```python
from build123d import *

# Parameters (mm, degrees)
SKETCH1_W           = 32
SKETCH1_H           = 15
BOSS_EXTRUDE1_DEPTH = 10
SKETCH2_R           = 2.5
BOSS_EXTRUDE2_DEPTH = 2
SKETCH3_W           = 30
SKETCH3_H           = 13
CUT_EXTRUDE1_DEPTH  = 9
SKETCH4_R           = 3.5
SKETCH4_R_2         = 3
BOSS_EXTRUDE3_DEPTH = 9
BOSS_EXTRUDE4_DEPTH = 7


with BuildPart() as part:
    # Sketch1 → Boss-Extrude1 (new body)
    with BuildSketch(Plane(origin=(0, 0, 0), x_dir=(1, 0, 0), z_dir=(0, 1, 0))):
        Rectangle(SKETCH1_W, SKETCH1_H)
    extrude(amount=BOSS_EXTRUDE1_DEPTH)

    # Sketch2 → Boss-Extrude2 (add)
    with BuildSketch(Plane(origin=(0, 10, 0), x_dir=(1, 0, 0), z_dir=(0, 1, 0))):
        with Locations((-12, -3.5)):
            Circle(SKETCH2_R)
        with Locations((-4, -3.5)):
            Circle(SKETCH2_R)
        with Locations((4, -3.5)):
            Circle(SKETCH2_R)
        with Locations((12, -3.5)):
            Circle(SKETCH2_R)
        with Locations((12, 3.5)):
            Circle(SKETCH2_R)
        with Locations((4, 3.5)):
            Circle(SKETCH2_R)
        with Locations((-4, 3.5)):
            Circle(SKETCH2_R)
        with Locations((-12, 3.5)):
            Circle(SKETCH2_R)
    extrude(amount=BOSS_EXTRUDE2_DEPTH)

    # Sketch3 → Cut-Extrude1 (cut)
    with BuildSketch(Plane.XZ):
        Rectangle(SKETCH3_W, SKETCH3_H)
    extrude(amount=-CUT_EXTRUDE1_DEPTH, mode=Mode.SUBTRACT)

    # Sketch4 → Boss-Extrude3 (add)
    with BuildSketch(Plane.XZ.offset(-9)):
        Circle(SKETCH4_R)
        Circle(SKETCH4_R_2, mode=Mode.SUBTRACT)
        with Locations((8, 0)):
            Circle(SKETCH4_R)
        with Locations((8, 0)):
            Circle(SKETCH4_R_2, mode=Mode.SUBTRACT)
        with Locations((-8, 0)):
            Circle(SKETCH4_R)
        with Locations((-8, 0)):
            Circle(SKETCH4_R_2, mode=Mode.SUBTRACT)
    extrude(amount=BOSS_EXTRUDE3_DEPTH)

    # Sketch5 → Boss-Extrude4 (add)
    with BuildSketch(Plane.XZ.offset(-9)):
        with BuildLine():
            Line((-0.272235441, -6.5), (0.272235441, -6.5))
            Line((0.272235441, -6.5), (0.272235441, -3.48939649))
            ThreePointArc((0.272235441, -3.48939649), (0, -3.5), (-0.272235441, -3.48939649))
            Line((-0.272235441, -3.48939649), (-0.272235441, -6.5))
        make_face()
        with BuildLine():
            Line((-0.272235441, 6.5), (0.272235441, 6.5))
            Line((0.272235441, 6.5), (0.272235441, 3.48939649))
            ThreePointArc((0.272235441, 3.48939649), (0, 3.5), (-0.272235441, 3.48939649))
            Line((-0.272235441, 3.48939649), (-0.272235441, 6.5))
        make_face()
    extrude(amount=BOSS_EXTRUDE4_DEPTH)


solid = part.part
```
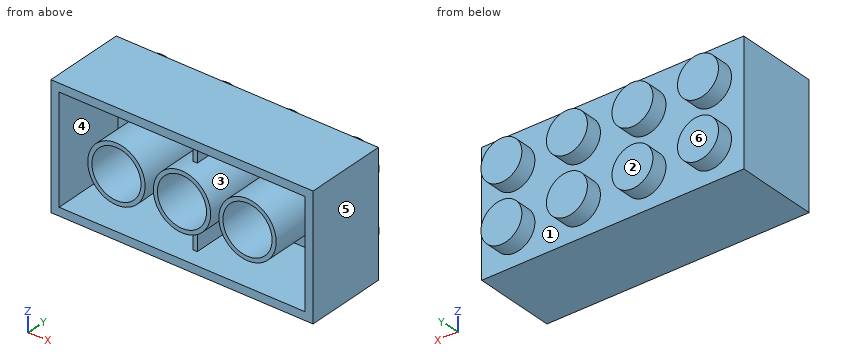
Geometry check sheet. Reference: the model listing, model coordinates, mm. Face numbers are marked on the shaded views. A direction names the side the tool comes from. Give positions to 0.01 mm unless a question says otherwise; leave off trailing zeros. Order: outer loops, then holes, each group sorted by start corner. A loop starts at its lowest first (then second) coordinate and runs counter-clockwise, first axis right, second up. Notation, with made-up numbers: (-32.75, -12.5) - (-5.75, -12.5) arc R31 ccw to (-5.75, 24.5) - close; hole circle Ø3 at (32, 35.5). An arc over 180 degrees is marked (long way). Answer in a Markdown table with one row per item. Add a question column.
Q1. Cross-section at C-C, the plane x = 8. Enter the section's corners in (y, z), then the cut area to 3 significant figures.
Q2. Material ranges on probe 1 along Z at (x, y) = (-8, 5.75); probe 2 along X at (y, z) = (3.75, 4.25); probe 3 along X at (y, z) = (11, 4), recorded low to high. Write a range as from..to.
Q3. Mould release check, pull along X, two halves, no side actions. Record for the marked faces 4, 5 and 6: pulls with the +X half, pulls with the -X half, needs draft (parallel to the pull), parting line crosses it, or undercut.
Q4. Cross-section at A-A, the plane y = 2.5. Enter the section's corners in (x, z), then the cut area to 3 significant figures.
Q5. Gauge pin test, flat ends, axial feed: pin 1 (0.6 mm diameter, centred on x = 0, z = -5, fed in from -Y); pin 2 (3 mm diameter, centred on x = -9, z = -3, fed in from +Y); pin 3 (1.8 mm diameter, centred on x = 8.5, z = -1, fed in from -Y); pin 4 (2 mm diameter, centred on x = 7, z = 5.5, fed in from +Y). Record the tip position at first contact, or that the pin passes through.
Q6. Cross-section at D-D, the plane x = 12. Enter the section's corners in (y, z), then the cut area to 3 significant figures.
Q7. Tool access check on the marked faces 1, 2 and 3. Record the directions out of +Z, -Z, +X, -X, +Y, -Y that give a thin tool (end or side, any length) a straight path to the whole face; none if there is none.
Check values:
| question | item | result |
|---|---|---|
| 1 | outline | (0, -7.5) - (10, -7.5) - (10, 7.5) - (0, 7.5) - (0, 6.5) - (9, 6.5) - (9, 3.5) - (0, 3.5) - (0, 3) - (9, 3) - (9, -3) - (0, -3) - (0, -3.5) - (9, -3.5) - (9, -6.5) - (0, -6.5) - close |
| 1 | area | 42.0 mm^2 |
| 2 | probe 1 | z = -7.5..-6.5, -3.5..-3, 3..3.5, 6.5..7.5 |
| 2 | probe 2 | x = -16..-15, -0.27..0.27, 15..16 |
| 2 | probe 3 | x = -14.45..-9.55, -6.45..-1.55, 1.55..6.45, 9.55..14.45 |
| 3 | face 4 | undercut |
| 3 | face 5 | pulls with the +X half |
| 3 | face 6 | needs draft |
| 4 | outline | (-16, -7.5) - (16, -7.5) - (16, 7.5) - (-16, 7.5) - close; circle Ø7 at (-8, 0); circle Ø7 at (8, 0); hole (-15, -6.5) - (-0.27, -6.5) - (-0.27, -3.49) arc R3.5 cw to (-0.27, 3.49) - (-0.27, 6.5) - (-15, 6.5) - close; hole circle Ø6 at (-8, 0); hole circle Ø6 at (0, 0); hole (0.27, -6.5) - (15, -6.5) - (15, 6.5) - (0.27, 6.5) - (0.27, 3.49) arc R3.5 cw to (0.27, -3.49) - close; hole circle Ø6 at (8, 0) |
| 4 | area | 124 mm^2 |
| 5 | pin 1 | stops at y = 2 |
| 5 | pin 2 | stops at y = 12 |
| 5 | pin 3 | stops at y = 9 |
| 5 | pin 4 | stops at y = 10 |
| 6 | outline | (0, -7.5) - (10, -7.5) - (10, -6) - (12, -6) - (12, -1) - (10, -1) - (10, 1) - (12, 1) - (12, 6) - (10, 6) - (10, 7.5) - (0, 7.5) - (0, 6.5) - (9, 6.5) - (9, -6.5) - (0, -6.5) - close |
| 6 | area | 53.0 mm^2 |
| 7 | face 1 | +Y |
| 7 | face 2 | +Z, -Z, +X, -X, +Y |
| 7 | face 3 | -Y |
